The figure shows three views and two pictorial views of one solid part (mm, origin at its lowest corner). Answer the questions. Coordinates: 2 decimals unless noted, no trailing zeros. Order: outer loops, then holes, each group sorted by start corner. A loop starts at its lowest first (then second) coordinate and runs counter-clockwise, first axis right, second up. Notation, with made-up numbers: (59, 21) - (114, 21) arc R20 ccw to (114, 58) - close; hole circle Ø1 at (78.5, -28). An arc over 180 degrees is marked (long way). Use one line per item in the form item = value.
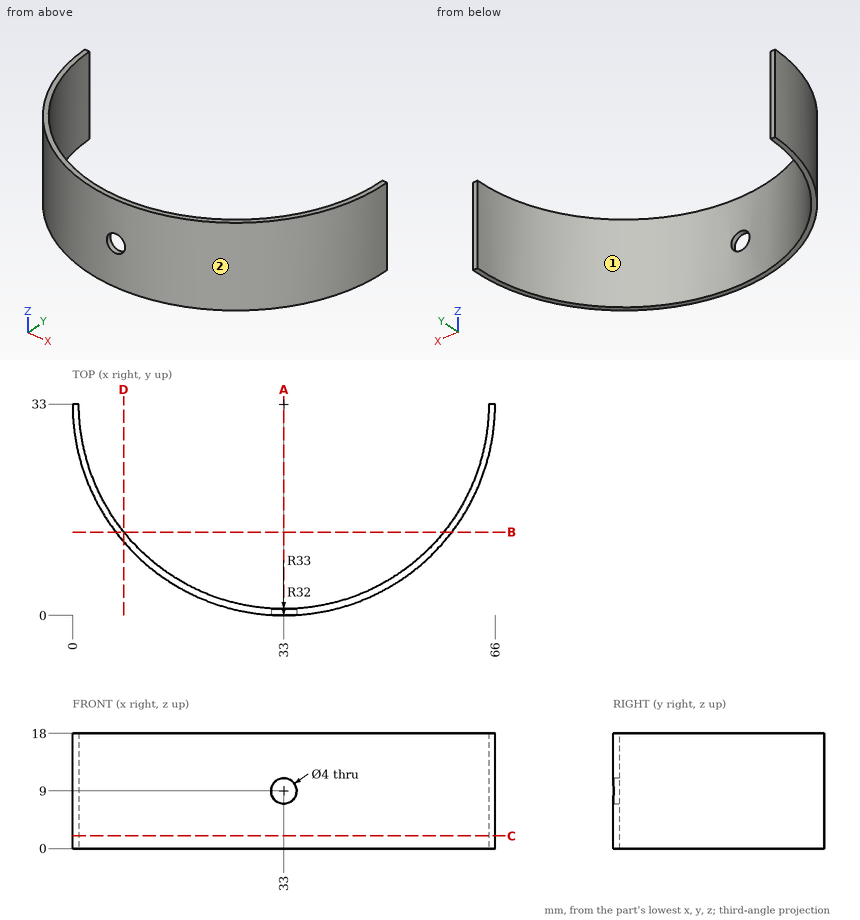
(1) Section D-D, the plane x = 8 is taken. Write down the section's boundary in (y, z).
Answer list:
outline = (11.46, 0) - (13.03, 0) - (13.03, 18) - (11.46, 18) - close
(2) The mould has two halves that part along X. Classify the marked faces 1 and 2: +X half, -X half, draft (parallel to the pull), parting line (faces both ways), or undercut.
Answer list:
face_1 = undercut
face_2 = parting line
(3) Section B-B, the plane y = 13 is taken. Write down the section's boundary in (x, z).
Answer list:
outline = (6.75, 0) - (8.02, 0) - (8.02, 18) - (6.75, 18) - close; (57.98, 0) - (59.25, 0) - (59.25, 18) - (57.98, 18) - close
(4) Straight lines are drawn through the part: L1, parallel to X at y = 28, z = 3.75; L2, parallel to X at y = 8.5, z = 3.5; L3, parallel to Y at x = 42.5, z = 14.75. For each, find the intervals that lie inside material, in ascending order.
Answer list:
L1 = 0.38 to 1.39, 64.61 to 65.62
L2 = 10.89 to 12.41, 53.59 to 55.11
L3 = 1.4 to 2.44
(5) Section A-A, the plane x = 33 is taken. Write down the section's boundary in (y, z), then the cut area to 3 significant figures.
Answer list:
outline = (0, 0) - (1, 0) - (1, 7) - (0, 7) - close; (0, 11) - (1, 11) - (1, 18) - (0, 18) - close
area = 14.0 mm2
(6) Given pin 1 Ø5 at (x, z) = (39.5, 2.5) entering from +Y; pin 2 Ø10 at (y, z) = (25, 5.5) entering from -X; pin 3 Ø1.5 at (y, z) = (27.5, 4.5) entering from +X, each flat-ended and moving along its own axis, determine where each tip first touches the part or whether it passes through.
Answer list:
pin_1 = 2.29
pin_2 = 0.14
pin_3 = 65.66
(7) Section C-C, the plane z = 2 is taken. Write down the section's boundary in (x, y).
Answer list:
outline = (0, 33) arc R33 ccw to (66, 33) - (65, 33) arc R32 cw to (1, 33) - close
